For this review, use the dimensioned drawing (mm, ordinates from the lowest corner) and the shaded views. A direction names the side the tool comes from. Round coordinates to 2 decimals unless told otherwise and drop trailing zeros. Write each loop counter-clockwise with the first axis right and the second up, starting at its lowest first coordinate (ties: lowest second). Pieces come first, ordered by that corner, then holes.
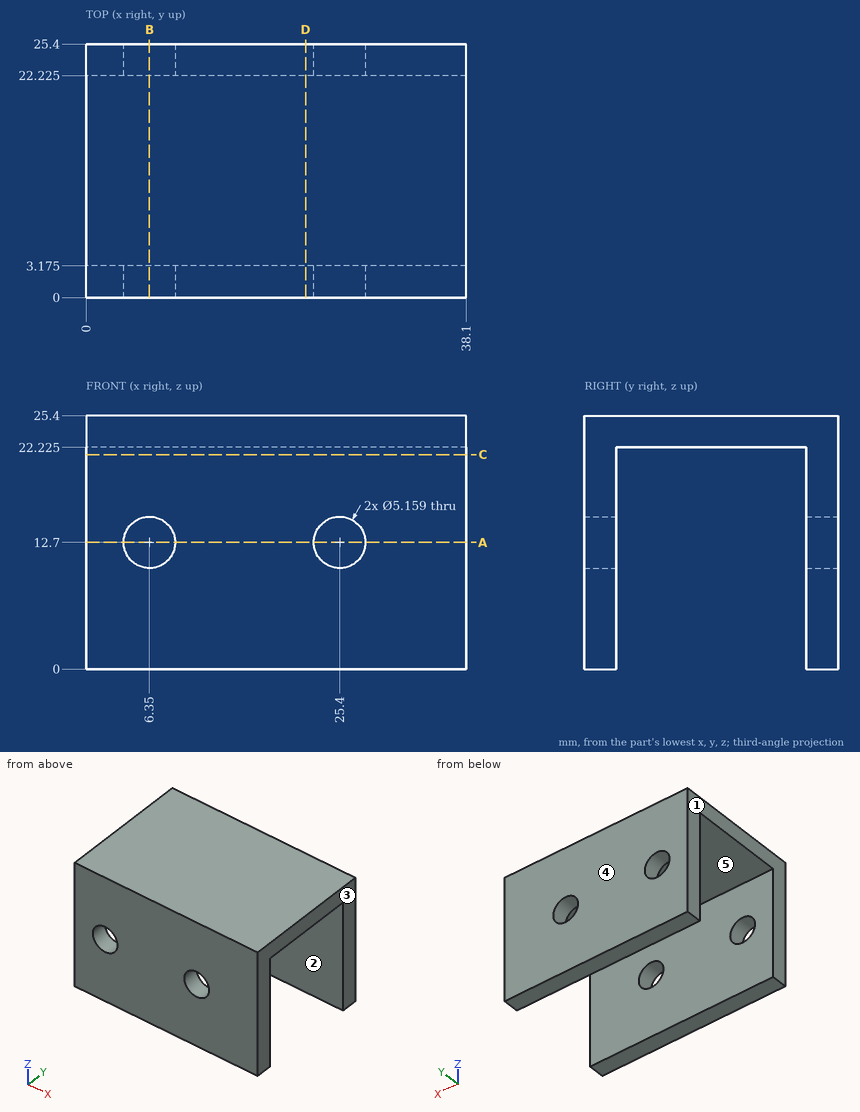
(1) We need section A-A, the plane z = 12.7. Give the boundary of the cut face in (x, y) (1 decimal).
Geometry check:
outline: (0, 0) - (3.8, 0) - (3.8, 3.2) - (0, 3.2) - close; (0, 22.2) - (3.8, 22.2) - (3.8, 25.4) - (0, 25.4) - close; (8.9, 0) - (22.8, 0) - (22.8, 3.2) - (8.9, 3.2) - close; (8.9, 22.2) - (22.8, 22.2) - (22.8, 25.4) - (8.9, 25.4) - close; (28, 0) - (38.1, 0) - (38.1, 3.2) - (28, 3.2) - close; (28, 22.2) - (38.1, 22.2) - (38.1, 25.4) - (28, 25.4) - close
(2) We need section C-C, the plane z = 21.5. Give the boundary of the cut face in (x, y) (1 decimal).
Geometry check:
outline: (0, 0) - (38.1, 0) - (38.1, 3.2) - (0, 3.2) - close; (0, 22.2) - (38.1, 22.2) - (38.1, 25.4) - (0, 25.4) - close
(3) For the marked faces 1 and 2, list the 3-axis set-ups (+Z, -Z, +X, -X, +Y, -Y) from which the entire face can be reached by the end or side of a thin tool; tool diameter is ignored.
Geometry check:
face 1: +Z, -Z, -X, +Y, -Y
face 2: -Z, +X, -X
(4) For pin 1 Ø4.5 at (x, z) = (6.35, 12.7) entering from +Y; pin 2 Ø3 at (x, y) = (22.5, 19.5) entering from -Z (3 decimals), all flat-tipped, find the tip position at first contact; note any pin that passes through.
Geometry check:
pin 1: passes through
pin 2: stops at z = 22.225
(5) Mouldability with a two-part tool opening along Y and no side actions: class the marked faces 3, 4 and 5 as pulls with the +Y half, pulls with the -Y half, needs draft (parallel to the pull), parting line crosses it, or undercut.
Geometry check:
face 3: needs draft
face 4: pulls with the +Y half
face 5: undercut
(6) We need section D-D, the plane x = 22. Give the boundary of the cut face in (y, z) (1 decimal), and give its area (3 significant figures).
Geometry check:
outline: (0, 0) - (3.2, 0) - (3.2, 22.2) - (22.2, 22.2) - (22.2, 0) - (25.4, 0) - (25.4, 25.4) - (0, 25.4) - close
area: 222 mm2
(7) For line 1 along X through (y, z) = (23.25, 12.7); line 2 along Z through (x, y) = (25.4, 1.6); line 3 along Y through (x, z) = (15.5, 17.5) (1 decimal), list the stretches that pass through material, from the lowest coordinate up.
Geometry check:
line 1: x = 0 to 3.77, 8.93 to 22.82, 27.98 to 38.1
line 2: z = 0 to 10.12, 15.28 to 25.4
line 3: y = 0 to 3.2, 22.2 to 25.4
(8) We need section B-B, the plane x = 6.35. Give the boundary of the cut face in (y, z) (1 decimal), and give its area (3 significant figures).
Geometry check:
outline: (0, 0) - (3.2, 0) - (3.2, 10.1) - (0, 10.1) - close; (0, 15.3) - (3.2, 15.3) - (3.2, 22.2) - (22.2, 22.2) - (22.2, 15.3) - (25.4, 15.3) - (25.4, 25.4) - (0, 25.4) - close; (22.2, 0) - (25.4, 0) - (25.4, 10.1) - (22.2, 10.1) - close
area: 189 mm2
